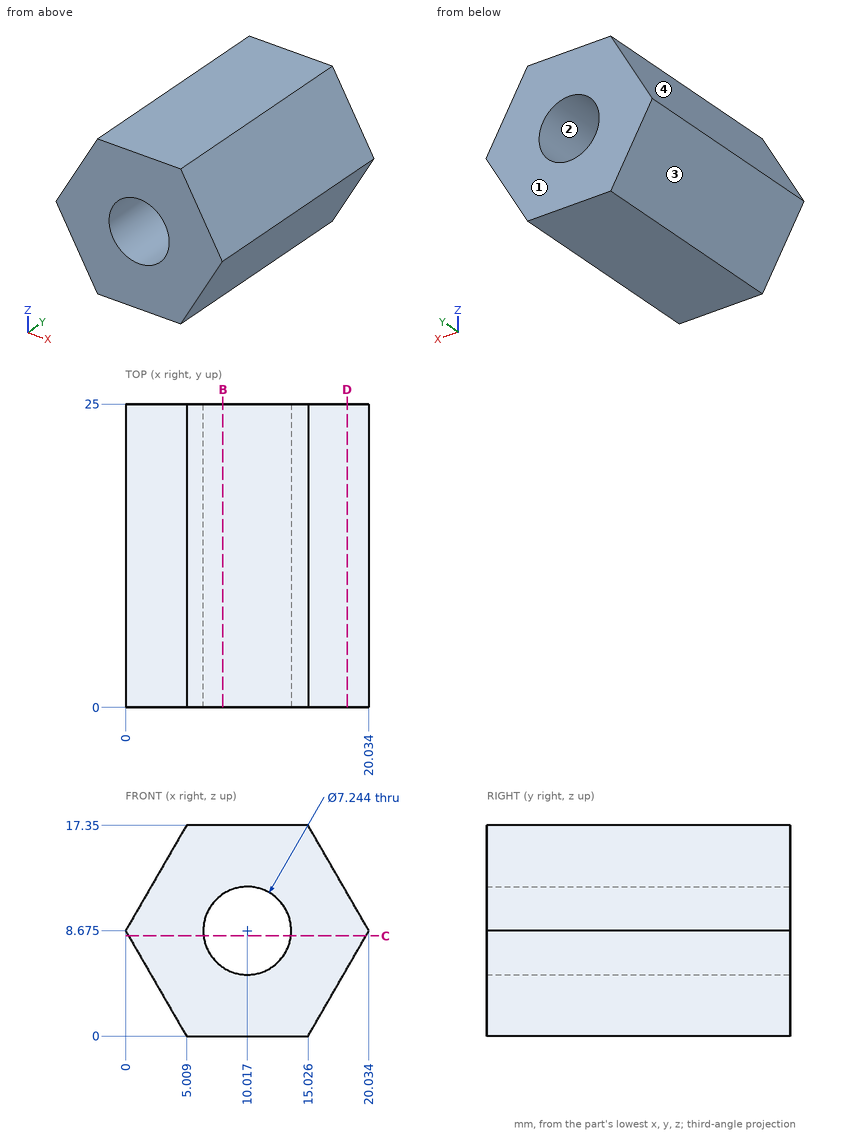
Study the drawing (mm; zero at the part's minimum x, y, z) and answer. Coordinates: 2 decimals unless noted, no trailing zeros. Write each loop counter-clockwise with the first axis right and the second up, starting at its lowest first coordinate (ties: lowest second). Pieces come first, ordered by that corner, then holes. Notation, with made-up numbers: (-32.75, 34) - (19.25, 34) arc R4 ccw to (19.25, 39) - close; hole circle Ø6 at (54.5, 6). An arc over 180 degrees is marked (long way). Return JSON: item names as keys, results as strings. Group by question number.
1. Determine the mould class of the marked faces 1, 2, 3 and 4 for opening direction Z: released by +Z, released by -Z, zero draft, split by the parting line, or undercut.
2. A cutting plane is placed at B-B, the plane x = 8. Determine the outline of the cut face in (y, z), plus the area to 3 significant figures.
3. Straight lines are drawn through the part: L1, parallel to Z at x = 9, y = 14; L2, parallel to X at y = 15.5, z = 5.5 (1 decimal); L3, parallel to Z at x = 9.5, y = 14. For each, find the intervals that lie inside material, in ascending order.
4. A cutting plane is placed at D-D, the plane x = 18.25. Determine the outline of the cut face in (y, z) (1 decimal).
5. Given pin 1 (2 mm diameter, centred on x = 2.5, y = 8.5, fed in from +Z) (1 decimal); pin 2 (1 mm diameter, centred on y = 7, z = 3.5, fed in from +X) (1 decimal); pin 3 (8 mm diameter, centred on y = 9.5, z = 15.5, fed in from +X), each flat-ended and moving along its own axis, determine where each tip first touches the part or whether it passes through.
6. A cutting plane is placed at C-C, the plane z = 8.25. Determine the outline of the cut face in (x, y) (1 decimal).
Ans:
{
 "1": {"face 1": "zero draft", "face 2": "undercut", "face 3": "released by -Z", "face 4": "released by +Z"},
 "2": {"outline": "(0, 0) - (25, 0) - (25, 5.67) - (0, 5.67) - close; (0, 11.68) - (25, 11.68) - (25, 17.35) - (0, 17.35) - close", "area": "283 mm²"},
 "3": {"L1": "0 to 5.2, 12.15 to 17.35", "L2": "1.8 to 8.3, 11.8 to 18.2", "L3": "0 to 5.09, 12.26 to 17.35"},
 "4": {"outline": "(0, 5.6) - (25, 5.6) - (25, 11.8) - (0, 11.8) - close"},
 "5": {"pin 1": "z = 14.7", "pin 2": "x = 17.3", "pin 3": "x = 18.4"},
 "6": {"outline": "(0.2, 0) - (6.4, 0) - (6.4, 25) - (0.2, 25) - close; (13.6, 0) - (19.8, 0) - (19.8, 25) - (13.6, 25) - close"}
}
